Can you work these out from the model? Positions are in its coordinate system, mm. A direction names the side the tool comes from. Round coordinates to 2 decimals unless told otherwise and drop trailing zeros. Write each loop counter-clockwise with the first axis right and the second up, starting at its lowest first coordinate (ties: lowest second). Pieces come first, ordered by that corner, then holes.
Q1. I'm going to push flat-ended pins straight in: pin 1 Ø2.5 at (y, z) = (25.5, 2) entering from +X; pin 2 Ø1.5 at (x, z) = (31.5, 1.5) entering from +Y; pin 3 Ø2.5 at (y, z) = (-25, 3) entering from -X. Where does each tip first touch, or does it pass through?
Q2. If we section it at B-B (y = -21): Please give me the cut outline in (x, z).
Q3. Please list where these lines run through material, in increasing order: line 1 along X through (y, z) = (30.5, 2.4); line 2 along Y through (x, z) = (3.5, 0.3); line 3 along X through (y, z) = (14.5, 2.35).
Q4. We'd pull the mould along X, two halves only. Please class faces 4 (the flat face through (30, -14, 2)), 5 (the flat face through (10, 31, 2)), 6 (the flat face through (-15, 28.5, 2)), 7 (the flat face through (32, -18.5, 3)): +X half, -X half, draft (parallel to the pull), parting line (faces both ways), or undercut.
Q5. For faces 1 (the flat face through (-25, 16, 2)), 2 (the flat face through (30, 25, 2)), 3 (the flat face through (30, 6, 2)), which set-ups out of +Z, -Z, +X, -X, +Y, -Y let a thin tool reach every point of the face, with its end or its side?
Q6. If we section it at C-C (x = 2.5): Please give me the cut outline in (y, z), plus the area to 3 significant figures.
from build123d import *

# Parameters (mm, degrees)
SKETCH_1_W             = 60
SKETCH_1_H             = 57
EXTRUDE_1_DEPTH        = 5
SKETCH_2_W             = 5
SKETCH_2_H             = 10
EXTRUDE_3_DEPTH        = 5
PATTERN_LINEAR_2_COUNT = 3
PATTERN_LINEAR_2_PITCH = 20
SKETCH_3_W             = 10
SKETCH_3_H             = 5
EXTRUDE_4_DEPTH        = 5
PATTERN_LINEAR_3_COUNT = 3
PATTERN_LINEAR_3_PITCH = 20
CUT_EXTRUDE_1_REACH    = 50.706
SKETCH_4_W             = 5
SKETCH_4_H             = 10
PATTERN_LINEAR_4_COUNT = 3
PATTERN_LINEAR_4_PITCH = 20


with BuildPart() as part:
    # 스케치1 → 보스-돌출1 (new body)
    with BuildSketch(Plane.XY):
        Rectangle(SKETCH_1_W, SKETCH_1_H)
    extrude(amount=EXTRUDE_1_DEPTH)

    # 스케치2 → 보스-돌출3 (add)
    with BuildSketch(Plane.XY.offset(5)):
        with Locations((32.5, -23.5)):
            Rectangle(SKETCH_2_W, SKETCH_2_H)
    extrude_3 = extrude(amount=-EXTRUDE_3_DEPTH)

    # 선형 패턴2: 보스-돌출3 ×3
    with Locations(*[(0, i * PATTERN_LINEAR_2_PITCH, 0) for i in range(1, PATTERN_LINEAR_2_COUNT)]):
        add(extrude_3)

    # 스케치3 → 보스-돌출4 (add)
    with BuildSketch(Plane(origin=(0, 0, 0), x_dir=(-1, 0, 0), z_dir=(0, 0, -1))):
        with Locations((25, 31)):
            Rectangle(SKETCH_3_W, SKETCH_3_H)
    extrude_4 = extrude(amount=-EXTRUDE_4_DEPTH)

    # 선형 패턴3: 보스-돌출4 ×3
    with Locations(*[(i * PATTERN_LINEAR_3_PITCH, 0, 0) for i in range(1, PATTERN_LINEAR_3_COUNT)]):
        add(extrude_4)

    # 스케치4 → 컷-돌출1 (cut, up to next)
    with BuildSketch(Plane(origin=(0, 0, 0), x_dir=(-1, 0, 0), z_dir=(0, 0, -1)), mode=Mode.PRIVATE) as cut_extrude_1_sk1:
        with Locations((27.5, -23.5)):
            Rectangle(SKETCH_4_W, SKETCH_4_H)
    cut_extrude_1_tool1 = extrude(cut_extrude_1_sk1.sketch, amount=-CUT_EXTRUDE_1_REACH, mode=Mode.PRIVATE) & part.part
    cut_extrude_1 = cut_extrude_1_tool1.solids().sort_by_distance((-27.5, -23.5, 0))[0]
    add(cut_extrude_1, mode=Mode.SUBTRACT)

    # 선형 패턴4: 컷-돌출1 ×3
    with Locations(*[(0, i * PATTERN_LINEAR_4_PITCH, 0) for i in range(1, PATTERN_LINEAR_4_COUNT)]):
        add(cut_extrude_1, mode=Mode.SUBTRACT)


solid = part.part
A:
1. pin 1: stops at x = 30
1. pin 2: stops at y = 21.5
1. pin 3: stops at x = -25
2. outline: (-25, 0) - (35, 0) - (35, 5) - (-25, 5) - close
3. line 1: x = -30 to -20, -10 to 0, 10 to 20
3. line 2: y = -28.5 to 28.5
3. line 3: x = -25 to 35
4. face 4: +X half
4. face 5: undercut
4. face 6: undercut
4. face 7: draft
5. face 1: +Z, -Z, -X
5. face 2: +Z, -Z, +X, +Y
5. face 3: +Z, -Z, +X
6. outline: (-28.5, 0) - (28.5, 0) - (28.5, 5) - (-28.5, 5) - close
6. area: 285 mm2
